For this review, use the dimensioned drawing (mm, ordinates from the lowest corner) and the shaded views. Coordinates: 2 decimals unless noted, no trailing zeros. Write each loop counter-clockwise with the first axis right and the second up, starting at its lowest first coordinate (ties: lowest second). Pieces come first, ordered by that corner, then holes.
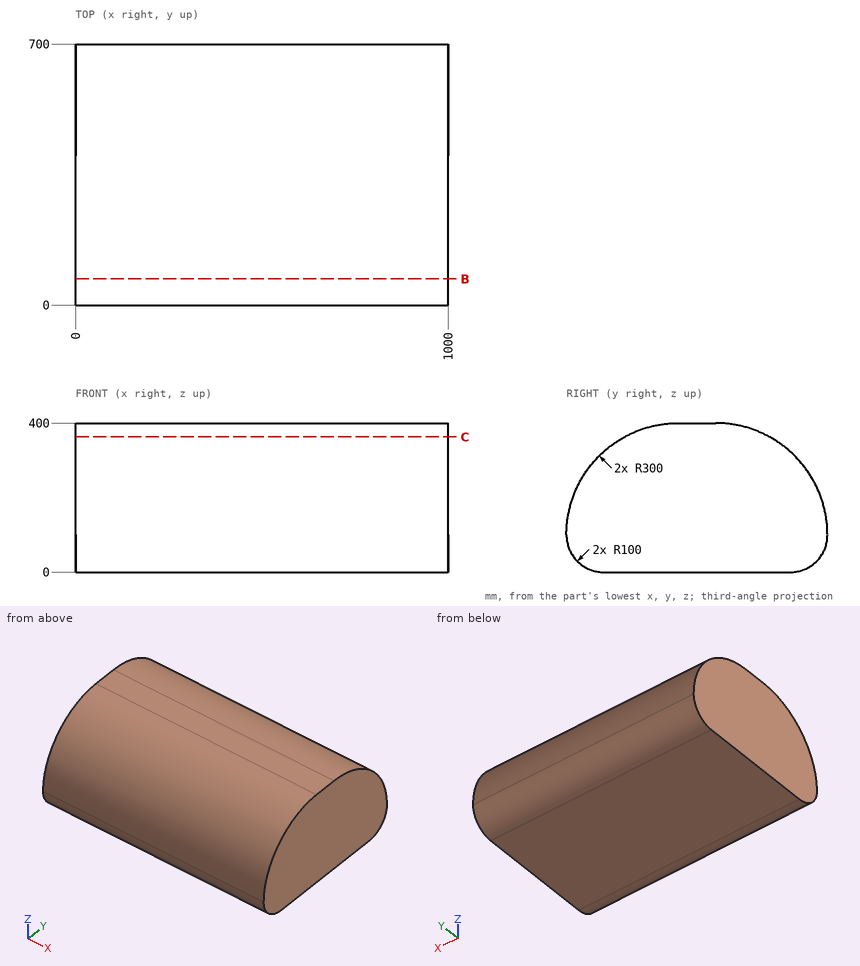
Item 1: For pin 1 (2 mm diameter, centred on x = 793.5, y = 467, fed in from +Z); pin 2 (12 mm diameter, centred on x = 598.5, y = 621, fed in from -Z); pin 3 (10 mm diameter, centred on x = 542.5, y = 192, fed in from -Z); pin 4 (12 mm diameter, centred on x = 678.5, z = 175, fed in from +Y), all flat-tipped, find the tip position at first contact; note any pin that passes through.
Solved:
pin 1: stops at z = 392.65
pin 2: stops at z = 1.13
pin 3: stops at z = 0
pin 4: stops at y = 691.96
Item 2: Take a section at C-C, the plane z = 363. Write out the cut boundary in (x, y), plus the area to 3 significant figures.
Solved:
outline: (0, 155.67) - (1000, 155.67) - (1000, 544.33) - (0, 544.33) - close
area: 389,000 mm2
Item 3: To check wall thickness, follow line 1 along Z through (x, y) = (874.5, 401); line 2 along Y through (x, z) = (218.5, 94); line 3 along Y through (x, z) = (314, 135). State the ranges of each line that lie inside material, in increasing order.
Solved:
line 1: z = 0 to 400
line 2: y = 0.18 to 699.82
line 3: y = 2.05 to 697.95
Item 4: Take a section at B-B, the plane y = 70.5. Write out the cut boundary in (x, z), plus the area to 3 significant figures.
Solved:
outline: (0, 4.45) - (1000, 4.45) - (1000, 293.21) - (0, 293.21) - close
area: 289,000 mm2
